Design review of the part built by this model. Coordinates are the model's own, in mm. A direction names the side the tool comes from. Give positions to 0.01 mm unless a question says otherwise; leave off trailing zeros. Write each loop counter-clockwise with the first axis right and the second up, starting at its lowest first coordinate (ties: lowest second). Pieces come first, ordered by that corner, then holes. Notation, with made-up numbers: (20, 74.5) -> (59, 74.5) arc R25 ccw to (59, 97.5) -> close; hole circle Ø3 at (8.25, -39). An arc over 180 degrees is marked (long way). Write each question's results on one line, items separated by ' | '. Start each with the question number.
(1) Clearance check with flat-ended pins moving along their axes: pin 1 (1.5 mm diameter, centred on y = 1, z = 7.5, fed in from -X); pin 2 (3 mm diameter, centred on y = 0, z = 66, fed in from -X); pin 3 (1 mm diameter, centred on y = 1, z = 66.5, fed in from +X). State where each tip first meets the part, or that it passes through.
(2) Take a section at B-B (z = 37). State the section outline as (x, y) points.
(3) To check wall thickness, follow probe 1 along X at (y, z) = (0.25, 51.5); probe 2 along Z at (x, y) = (-1.4, -2); probe 3 along Y at (x, z) = (-0.1, 30). State the ranges of each line that lie inside material, in increasing order.
(4) For faces 1 (the face through (-1, 0, 59)), 2 (the face through (0, 0, 0)), list the 3-axis set-ups (+Z, -Z, +X, -X, +Y, -Y) from which the entire face can be reached by the end or side of a thin tool; tool diameter is ignored.
(5) Take a section at A-A (y = 0). State the section outline as (x, z) points, plus the area to 3 significant figures.
from build123d import *

# Parameters (mm, degrees)
SKETCH1_R           = 3
BOSS_EXTRUDE1_DEPTH = 75
CHAMFER1_SIZE       = 0.5
CUT_EXTRUDE2_START  = -16
CUT_EXTRUDE2_DEPTH  = 16


with BuildPart() as part:
    # Sketch1 → Boss-Extrude1 (new body)
    with BuildSketch(Plane.XY):
        Circle(SKETCH1_R)
    extrude(amount=BOSS_EXTRUDE1_DEPTH)

    # Chamfer1
    chamfer1_edges = [part.edges().sort_by_distance(p)[0] for p in [
        (-3, 0, 0),
        (-3, 0, 75),
    ]]
    chamfer(chamfer1_edges, length=CHAMFER1_SIZE)

    # Sketch2 → Cut-Extrude2 (cut)
    with BuildSketch(Plane.XY.offset(75).offset(CUT_EXTRUDE2_START)):
        with BuildLine():
            Line((0, -3), (0, 3))
            ThreePointArc((0, 3), (-3, 0), (0, -3))
        make_face()
    extrude(amount=CUT_EXTRUDE2_DEPTH, mode=Mode.SUBTRACT)


solid = part.part
Report:
1) pin 1: x = -2.99 | pin 2: x = 0 | pin 3: x = 2.96
2) outline: circle Ø6 at (0, 0)
3) probe 1: -2.99 to 2.99 | probe 2: 0 to 59 | probe 3: -3 to 3
4) face 1: +Z, -X, +Y, -Y | face 2: -Z, +X, -X, +Y, -Y
5) outline: (-3, 0.5) -> (-2.5, 0) -> (2.5, 0) -> (3, 0.5) -> (3, 74.5) -> (2.5, 75) -> (0, 75) -> (0, 59) -> (-3, 59) -> close | area: 402 mm2
